Input: part model. Units: mm. Frame: model coordinates. A direction names the side the tool comes from. Give positions to 0.01 mm unless a question says otherwise; leave off trailing zeros. Write each loop counter-clockwise with the first axis right and the second up, starting at its lowest first coordinate (ties: lowest second). Pieces come first, ordered by that corner, then holes. Notation, with made-up numbers: (54.25, 14) -> (69.25, 14) arc R16 ccw to (69.25, 33) -> close; hole circle Ø8 at (-38, 11.5). An arc over 180 degrees is marked (long way). Answer as a JSON object with one key per item and string values. Group by question number.
from build123d import *


with BuildPart() as part:
    # Sweep1: sweep along a path in Sketch1
    with BuildLine(Plane(origin=(0, 0, 0), x_dir=(1, 0, 0), z_dir=(0, 1, 0))) as sweep1_path:
        Line((46.75, -25.25), (-46.75, -25.25))
        Line((-46.75, -25.25), (-46.75, 25.25))
        Line((-46.75, 25.25), (46.75, 25.25))
    # Sketch2 → Sweep1 (sweep)
    with BuildSketch(Plane(origin=(46.75, 0, 0), x_dir=(0, 0, -1), z_dir=(1, 0, 0))):
        Polygon((-25.25, 0.85), (-25.25, -0.85), (-22.25, -0.85), (-22.25, -5.85), (-28.25, -5.85), (-28.25, 14.15), (-22.25, 14.15), (-22.25, 0.85), align=None)
    sweep(path=sweep1_path.line, transition=Transition.RIGHT)


solid = part.part
1. Reachability of faces 1 (the face through (-7, 0.85, 23)), 2 (the face through (-2, 4, 28.25)), 3 (the face through (-43.75, -3, 0)) from +Z, -Z, +X, -X, +Y, -Y: full face, straight path, thin tool, end or side. Return the list, or none.
2. Section B-B (y = 9.25). Return the cut outline in (x, z).
3. Line query: line 1 (Z direction, x = 20, y = 11.5); line 2 (Y direction, x = -9, z = -23.5); line 3 (Z direction, x = 1, y = 0). Output: solid intervals per line, ascending.
4. Section C-C (z = -16). Return the cut outline in (x, y), plus the area to 3 significant figures.
5. Mould query, pull axis Z, two halves, no side actions, for faces 4 (the face through (1, -3, 22.25)), 5 (the face through (-1, 4, -28.25)), 6 (the face through (46.75, 4, 25)). Classes: pulls with the +Z half, pulls with the -Z half, needs draft (parallel to the pull), parting line crosses it, or undercut.
6. Contact query for flat-ended pins moving along their axis: pin 1 Ø2.5 at (y, z) = (-3, 6) entering from +X; pin 2 Ø25 at (x, z) = (-8.5, -2.5) entering from -Y. Output: stop coordinate, or through.
7. Section A-A (x = 7). Return the cut outline in (y, z).
Working result:
{
 "1": {"face 1": "+X", "face 2": "+Z, +X, -X, +Y, -Y", "face 3": "+X, +Y, -Y"},
 "2": {"outline": "(-49.75, -28.25) -> (46.75, -28.25) -> (46.75, -22.25) -> (-43.75, -22.25) -> (-43.75, 22.25) -> (46.75, 22.25) -> (46.75, 28.25) -> (-49.75, 28.25) -> close"},
 "3": {"line 1": "z = -28.25 to -22.25, 22.25 to 28.25", "line 2": "y = -5.85 to -0.85, 0.85 to 14.15", "line 3": "z = -28.25 to -25.25, 25.25 to 28.25"},
 "4": {"outline": "(-49.75, -5.85) -> (-43.75, -5.85) -> (-43.75, -0.85) -> (-46.75, -0.85) -> (-46.75, 0.85) -> (-43.75, 0.85) -> (-43.75, 14.15) -> (-49.75, 14.15) -> close", "area": "115 mm^2"},
 "5": {"face 4": "undercut", "face 5": "pulls with the -Z half", "face 6": "needs draft"},
 "6": {"pin 1": "stops at x = -43.75", "pin 2": "passes through"},
 "7": {"outline": "(-5.85, -28.25) -> (14.15, -28.25) -> (14.15, -22.25) -> (0.85, -22.25) -> (0.85, -25.25) -> (-0.85, -25.25) -> (-0.85, -22.25) -> (-5.85, -22.25) -> close; (-5.85, 22.25) -> (-0.85, 22.25) -> (-0.85, 25.25) -> (0.85, 25.25) -> (0.85, 22.25) -> (14.15, 22.25) -> (14.15, 28.25) -> (-5.85, 28.25) -> close"}
}
